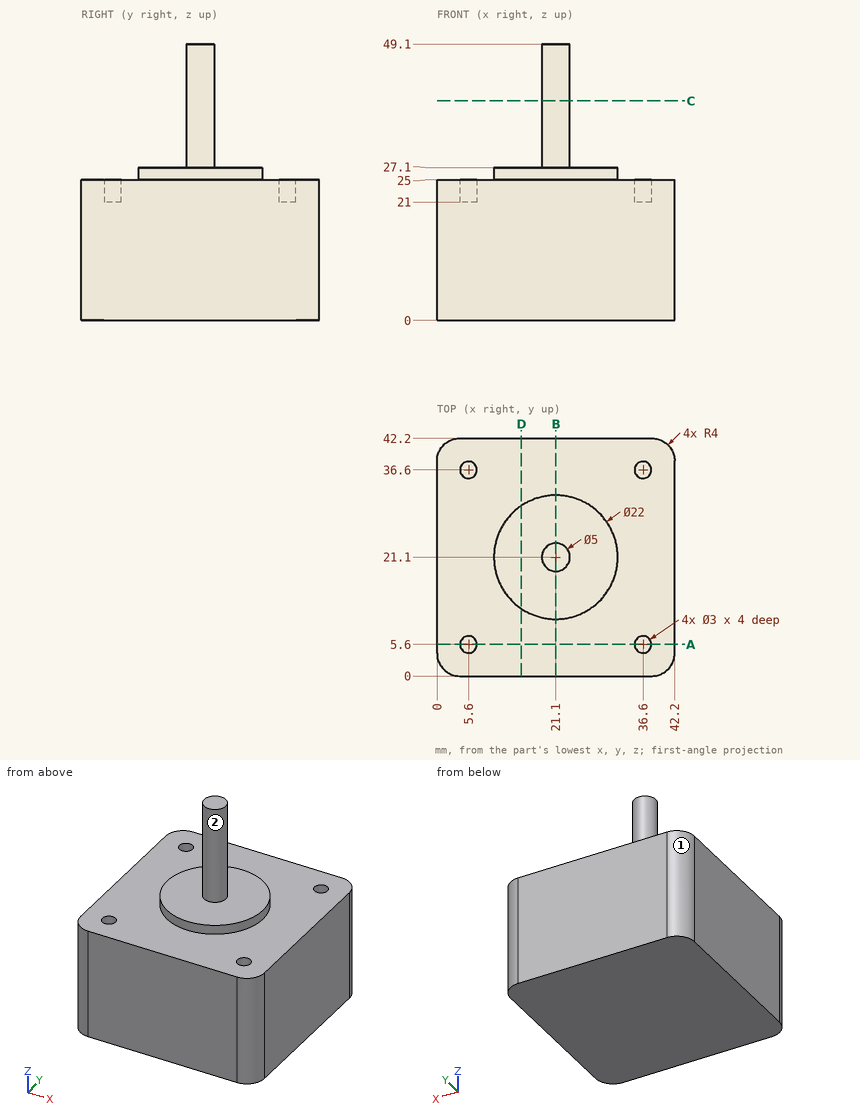
Here's the drawing with two shaded views (mm, measured from the low corner). I have some questions. A direction names the side the tool comes from. Coordinates: 2 decimals unless noted, no trailing zeros. Loops run counter-clockwise (first coordinate to the right, second up) from the corner with the lowest first, then second, coordinate; pieces in that order, holes last.
Item 1: Suppose I cut it at C-C (z = 39). Please give me the cut outline in (x, y).
Answers below:
outline: circle Ø5 at (21.1, 21.1)
Item 2: I'm going to push flat-ended pins straight in: pin 1 (3.5 mm diameter, centred on x = 5.6, y = 36.6, fed in from +Z); pin 2 (2 mm diameter, centred on y = 21.5, z = 31, fed in from -X); pin 3 (1.5 mm diameter, centred on x = 36, y = 5.5, fed in from +Z); pin 4 (2 mm diameter, centred on y = 16.5, z = 28.5, fed in from +X). Where does each tip first touch, or does it pass through?
Answers below:
pin 1: stops at z = 25
pin 2: stops at x = 18.6
pin 3: stops at z = 21
pin 4: passes through
Item 3: Suppose I cut it at D-D (x = 15). Please give me the cut outline in (y, z), then the cut area to 3 significant figures.
Answers below:
outline: (0, 0) - (42.2, 0) - (42.2, 25) - (30.25, 25) - (30.25, 27.1) - (11.95, 27.1) - (11.95, 25) - (0, 25) - close
area: 1,090 mm2
Item 4: Please list where these lines run through material, in increasing order: L1, parallel to Y at x = 36.6, z = 23.95; L2, parallel to Y at x = 36, z = 22.
Answers below:
L1: y = 0 to 4.1, 7.1 to 35.1, 38.1 to 42.2
L2: y = 0 to 4.23, 6.97 to 35.23, 37.97 to 42.2
Item 5: Suppose I cut it at A-A (y = 5.6). Please give me the cut outline in (x, z), then the cut area to 3 significant figures.
Answers below:
outline: (0, 0) - (42.2, 0) - (42.2, 25) - (38.1, 25) - (38.1, 21) - (35.1, 21) - (35.1, 25) - (7.1, 25) - (7.1, 21) - (4.1, 21) - (4.1, 25) - (0, 25) - close
area: 1,030 mm2
Item 6: Suppose I cut it at B-B (x = 21.1). Please give me the cut outline in (y, z).
Answers below:
outline: (0, 0) - (42.2, 0) - (42.2, 25) - (32.1, 25) - (32.1, 27.1) - (23.6, 27.1) - (23.6, 49.1) - (18.6, 49.1) - (18.6, 27.1) - (10.1, 27.1) - (10.1, 25) - (0, 25) - close
Item 7: Which directions (+Z, -Z, +X, -X, +Y, -Y) give clear straight access to the entire face, cutting with the end or side of a thin tool? Please do the marked faces 1 and 2.
Answers below:
face 1: +Z, -Z, -X, +Y
face 2: +Z
